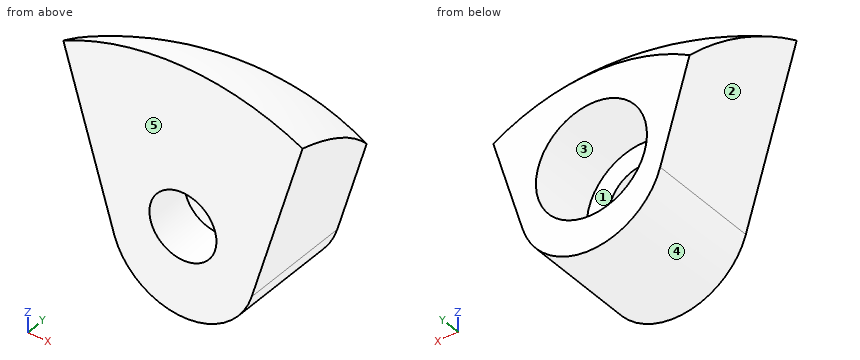
from build123d import *

# Parameters (mm, degrees)
CUT_EXTRUDE1_DEPTH = 8.493


with BuildPart() as part:
    # Sketch1 → Revolve1 (revolve)
    with BuildSketch(Plane.XY):
        with BuildLine():
            Line((0, 0), (19.05, 0))
            ThreePointArc((19.05, 0), (13.470384182, 13.470384182), (0, 19.05))
            Line((0, 19.05), (0, 0))
        make_face()
    revolve(axis=Axis((0, 19.05, 0), (0, -1, 0)))

    # SurfaceCut1
    split(bisect_by=Plane(origin=(0, 13.843, 0), x_dir=(-1, 0, 0), z_dir=(0, 1, 0)), keep=Keep.BOTTOM)

    # SurfaceCut2
    split(bisect_by=Plane(origin=(0, 6.35, 0), x_dir=(-1, 0, 0), z_dir=(0, 1, 0)), keep=Keep.TOP)

    # Sketch2 → Cut-Extrude1 (cut, through all)
    with BuildSketch(Plane(origin=(0, 6.35, 0), x_dir=(-1, 0, 0), z_dir=(0, 1, 0))):
        with BuildLine():
            Line((4.562115728, 4.846079058), (7.9375, 16.11136536))
            ThreePointArc((7.9375, 16.11136536), (0, -17.960512242), (-7.9375, 16.11136536))
            Line((-7.9375, 16.11136536), (-4.562115728, 4.846079058))
            ThreePointArc((-4.562115728, 4.846079058), (0, 1.450512242), (4.562115728, 4.846079058))
        make_face()
    extrude(amount=CUT_EXTRUDE1_DEPTH, mode=Mode.SUBTRACT)

    # Sketch4 → Cut-Revolve1 (revolve, cut)
    with BuildSketch(Plane(origin=(0, 0, 0), x_dir=(0, 0, -1), z_dir=(1, 0, 0))):
        Polygon((-7.419512242, 13.843), (-7.419512242, 6.35), (-5.197012242, 6.35), (-5.197012242, 9.398), (-3.736512242, 9.398), (-3.736512242, 13.843), align=None)
    revolve(axis=Axis((0, 6.35, 7.419512242), (0, 1, 0)), mode=Mode.SUBTRACT)


solid = part.part
Input: part model. Units: mm. Frame: model coordinates. Face numbers are marked on the shaded views. A direction names the side the tool comes from. Give positions to 0.01 mm unless a question says otherwise; leave off trailing zeros. Write each loop counter-clockwise with the first axis right and the second up, starting at its lowest first coordinate (ties: lowest second). Pieces come first, ordered by that corner, then holes. Notation, with made-up numbers: (28.5, -10.5) -> (77.5, -10.5) arc R19 ccw to (77.5, 10.5) -> close; hole circle Ø4 at (-24.75, 59.5). An arc over 180 degrees is marked (long way). Use one line per item in the form item = value. Start each with the question number.
1) Section query A-A on x = 0. Return the cut outline in (y, z).
2) Pin query (flat end, axial travel): pin 1 (3 mm diameter, centred on x = 5.5, y = 7, fed in from +Z); pin 2 (3 mm diameter, centred on y = 10, z = 13.5, fed in from +X); pin 3 (1 mm diameter, centred on x = -3.5, z = 13.5, fed in from +Y). Return the tip coordinate at first contact, or that it passes through.
3) Set-up query: the marked faces 1 and 2. Return all of +Z, -Z, +X, -X, +Y, -Y with unobstructed straight access to the full face (end or side cutting, diameter ignored); none if empty.
4) Ray query, probe 1 along X at (y, z) = (11.5, 8.5); probe 2 along Z at (x, y) = (0, 7); probe 3 along Z at (x, y) = (0, 7.85). Return the intervals inside material, ascending. Write a range as from..to.
5) Draft query along X for the marked faces 3, 4 and 5. Return one class per face: pulls with the +X half, pulls with the -X half, needs draft (parallel to the pull), parting line crosses it, or undercut.
6) Section query B-B on z = 9. Return the cut outline in (x, y), then the cut area to 3 significant figures.
7) Section query D-D on x = -3. Return the cut outline in (y, z), then the cut area to 3 significant figures.
8) Section query C-C on y = 13.25. Return the cut outline in (x, z) (1 decimal).
Outcome:
q1.outline = (6.35, 1.45) -> (13.84, 1.45) -> (13.84, 3.74) -> (9.4, 3.74) -> (9.4, 5.2) -> (6.35, 5.2) -> close; (6.35, 9.64) -> (9.4, 9.64) -> (9.4, 11.1) -> (13.84, 11.1) -> (13.84, 13.09) arc R19.05 ccw to (6.35, 17.96) -> close
q2.pin_1 = 17.47
q2.pin_2 = 7.55
q2.pin_3 = 13.49
q3.face_1 = +Y
q3.face_2 = -Z, -X, +Y, -Y
q4.probe_1 = -5.66..-3.52, 3.52..5.66
q4.probe_2 = 1.45..5.2, 9.64..17.72
q4.probe_3 = 1.45..5.2, 9.64..17.36
q5.face_3 = undercut
q5.face_4 = parting line crosses it
q5.face_5 = needs draft
q6.outline = (-5.81, 6.35) -> (-1.56, 6.35) -> (-1.56, 9.4) -> (-3.33, 9.4) -> (-3.33, 13.84) -> (-5.81, 13.84) -> close; (1.56, 6.35) -> (5.81, 6.35) -> (5.81, 13.84) -> (3.33, 13.84) -> (3.33, 9.4) -> (1.56, 9.4) -> close
q6.area = 47.9 mm^2
q7.outline = (6.35, 2.51) -> (13.84, 2.51) -> (13.84, 5.28) -> (9.4, 5.28) -> (9.4, 9.56) -> (13.84, 9.56) -> (13.84, 12.74) arc R18.81 ccw to (6.35, 17.71) -> close
q7.area = 79.5 mm^2
q8.outline = (-6.7, 11.9) -> (-4.6, 4.8) arc R4.8 ccw to (4.6, 4.8) -> (6.7, 11.9) arc R13.7 ccw to start; hole circle Ø7.4 at (0, 7.4)
